Here's the drawing with two shaded views (mm, measured from the low corner). I have some questions. A direction names the side the tool comes from. Coordinates: 2 decimals unless noted, no trailing zeros. Write each loop counter-clockwise with the first axis right and the second up, starting at its lowest first coordinate (ties: lowest second). Pieces come first, ordered by that corner, then holes.
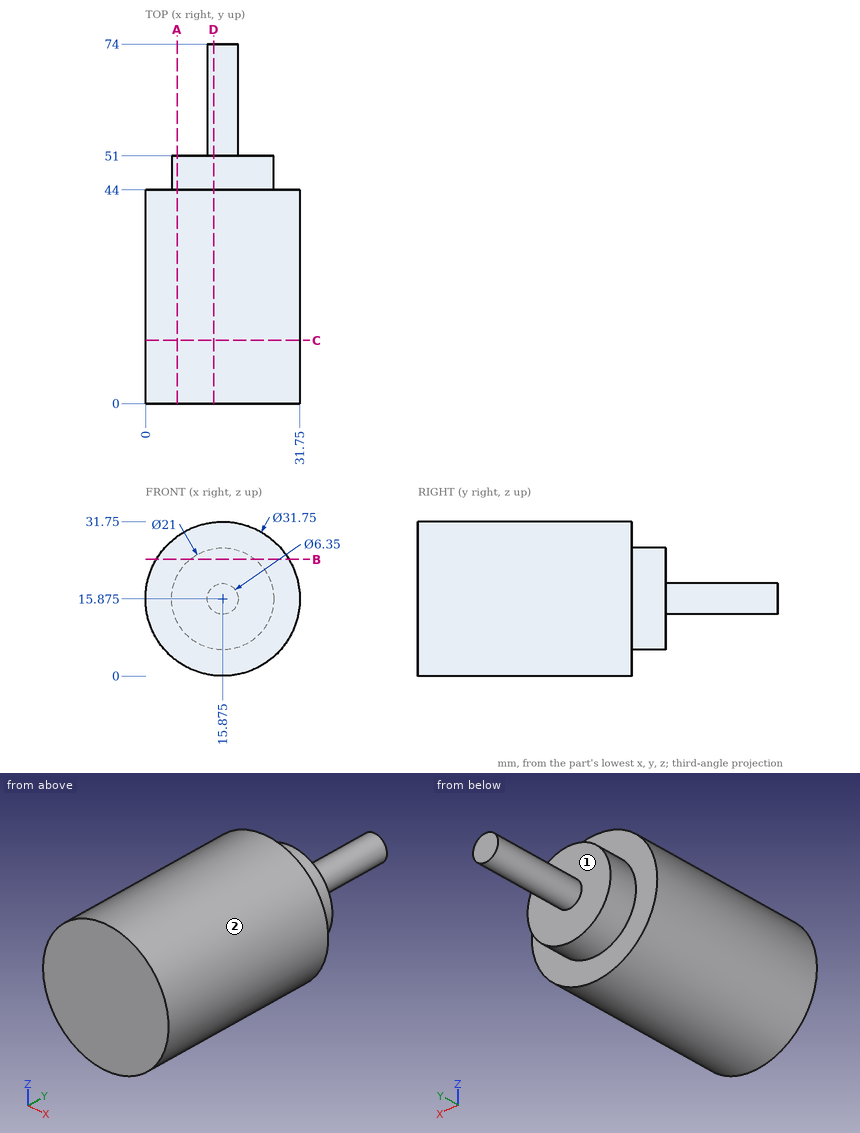
1. Please list where these lines run through material, in increasing order: line 1 along Y through (x, z) = (14.5, 27); line 2 along Y through (x, z) = (12.5, 25); line 3 along X through (y, z) = (22, 15.5).
Verdict:
line 1: y = 0 to 44
line 2: y = 0 to 51
line 3: x = 0 to 31.75
2. I want a section at D-D on x = 14. Please give me the cut outline in (y, z).
Verdict:
outline: (0, 0.11) - (44, 0.11) - (44, 5.54) - (51, 5.54) - (51, 13.31) - (74, 13.31) - (74, 18.44) - (51, 18.44) - (51, 26.21) - (44, 26.21) - (44, 31.64) - (0, 31.64) - close
3. I want a section at C-C on y = 13. Please give me the cut outline in (x, z) (3 decimals).
Verdict:
outline: circle Ø31.75 at (15.875, 15.875)
4. I want a section at A-A on x = 6.5. Please give me the cut outline in (y, z).
Verdict:
outline: (0, 3.06) - (44, 3.06) - (44, 11.15) - (51, 11.15) - (51, 20.6) - (44, 20.6) - (44, 28.69) - (0, 28.69) - close
5. On a 3-axis mill with a long thin cutter (end or side, diameter ignored), from which of +Z, -Z, +X, -X, +Y, -Y can I reach the whole of each face in a straight line? I mean the marked faces 1 and 2. Say none if no direction works.
Verdict:
face 1: +Y
face 2: +Y, -Y
6. I want a section at B-B on z = 24. Please give me the cut outline in (x, y).
Verdict:
outline: (2.24, 0) - (29.51, 0) - (29.51, 44) - (22.53, 44) - (22.53, 51) - (9.22, 51) - (9.22, 44) - (2.24, 44) - close
7. For pin 1 (12 mm diameter, centred on y = 18, z = 19.5, fed in from +X); pin 2 (5 mm diameter, centred on x = 12, z = 5, fed in from +Y); pin 3 (1 mm diameter, centred on y = 23, z = 22.5, fed in from -X); pin 4 (2 mm diameter, centred on x = 27.5, z = 26.5, fed in from +Y), each with a flat end and sliding along its axis, tell me the tip position at first contact or that it passes through.
Verdict:
pin 1: stops at x = 31.75
pin 2: stops at y = 51
pin 3: stops at x = 1.23
pin 4: stops at y = 44
